Here's how the part is built. I have some questions about the finished solid (model axes, mm). Give positions to 0.01 mm unless a question says otherwise; leave off trailing zeros. Write each loop counter-clockwise with the first axis right and the second up, starting at its lowest first coordinate (ties: lowest second). Pieces come first, ordered by that corner, then holes. Notation, with made-up numbers: (58.5, 51.5) -> (73.5, 51.5) arc R21 cw to (73.5, 62.5) -> close; hole circle Ø10 at (64, 37). An arc over 180 degrees is marked (long way). Use one line per item in the form item = value.
Autodesk Inventor part; units mm, degrees
ref_plane "作業平面1" through (0, 8, 0) normal (0, -0.7881, 0.6155) x (1, 0, 0)
ref_plane "作業平面2" through (0, -5, -3.1241) normal (0, -0.977, 0.2132) x (-0.3818, -0.1971, -0.903)
ref_plane "作業平面3" through (-5, 8, -6) normal (0, 0, 1) x (1, 0, 0)
sketch "スケッチ1" plane through (0, 0, 0) normal (0, 1, 0) x (-1, 0, 0)
  line L0 (-17.5, -21) -> (0, 0)
  line L1 (0, 0) -> (17.5, -21)
  line L2 (17.5, -21) -> (17.5, -41)
  line L3 (17.5, -41) -> (0, -50)
  line L4 (0, -50) -> (-17.5, -41)
  line L5 (-17.5, -41) -> (-17.5, -21)
  line L6 (0, -60) -> (0, 10)
  line L7 (24.5, 0) -> (-24.5, 0)
  dimension "d0" = 50
  dimension "d12" = 35
  dimension "d13" = 20
  dimension "d14" = 21
extrude "押し出し1" add sketch "スケッチ1" along normal blind 18
chamfer "面取り1" distance 5 distance2 10 6 edges at (8.75, 18, -10.5) (17.5, 18, -31) (8.75, 18, -45.5) (-8.75, 18, -45.5) (-17.5, 18, -31) (-8.75, 18, -10.5) measured on face at (0, 18, -30.6667)
extrude "押し出し2" add sketch "スケッチ1" against normal blind 5
ref_plane "作業平面1" through (0, 8, 0) normal (0, -0.7881, 0.6155) x (1, 0, 0)
sketch "スケッチ2" plane through (0, 8, 0) normal (0, -0.7881, 0.6155) x (1, 0, 0)
  line L0 (0, 0) -> (17.5, -16.5503)
  line L1 (-17.5, -16.5503) -> (0, 0)
  line L2 (-5, -4.7287) -> (-5, -4.7287)
  line L3 (-5, -4.7287) -> (5, -4.7287)
  line L4 (13.3346, -12.611) -> (5, -4.7287)
  line L5 (-5, -4.7287) -> (-23.6413, -26.9446)
  line L6 (5, -4.7287) -> (18.7173, -21.0763)
  line L7 (-23.6413, -26.9446) -> (-26.2109, -24.7885)
  line L8 (-26.2109, -24.7885) -> (-17.5, -16.5503)
  line L9 (17.5, -16.5503) -> (23.8178, -21.8516)
  line L10 (23.8178, -21.8516) -> (18.7173, -21.0763)
  point P0 (0, -4.9243)
  dimension "d9" = 10
  dimension "d25" = 130
  dimension "d26" = 130
extrude "押し出し3" cut sketch "スケッチ2" against normal through all
chamfer "面取り2" distance 2 distance2 8 6 edges at (-8.75, -5, -10.5) (-17.5, -5, -31) (-8.75, -5, -45.5) (8.75, -5, -45.5) (17.5, -5, -31) (8.75, -5, -10.5) measured on face at (0, -5, -30.6667)
sketch "スケッチ3" plane through (0, -5, 0) normal (0, -1, 0) x (1, 0, 0)
  line L0 (0, -3.1241) -> (15.5, -21.7241)
  line L1 (-15.5, -21.7241) -> (0, -3.1241)
  line L2 (-15.5, -39.7796) -> (-15.5, -21.7241)
  line L3 (0, -47.751) -> (-15.5, -39.7796)
  line L4 (15.5, -39.7796) -> (0, -47.751)
  line L5 (15.5, -21.7241) -> (15.5, -39.7796)
  point P0 (0, 0)
extrude "押し出し4" add sketch "スケッチ3" along normal blind 8
ref_plane "作業平面2" through (0, -5, -3.1241) normal (0, -0.977, 0.2132) x (-0.3818, -0.1971, -0.903)
sketch "スケッチ4" plane through (0, -5, -3.1241) normal (0, -0.977, 0.2132) x (-0.3818, -0.1971, -0.903)
  line L0 (80, -28.4848) -> (-10, -28.4848)
  line L1 (-10, -28.4848) -> (-10, 40)
  line L2 (-10, 40) -> (80, 40)
  line L3 (80, 40) -> (80, -28.4848)
  point P0 (-3.8064, -1.5725)
extrude "押し出し5" cut sketch "スケッチ4" along normal through all
ref_plane "作業平面3" through (-5, 8, -6) normal (0, 0, 1) x (1, 0, 0)
sketch "スケッチ5" plane through (-5, 8, -6) normal (0, 0, 1) x (1, 0, 0)
  line L0 (-30, 20) -> (40, 20)
  line L1 (40, 20) -> (40, -30)
  line L2 (40, -30) -> (-30, -30)
  line L3 (-30, -30) -> (-30, 20)
  point P0 (5, -8)
extrude "押し出し6" cut sketch "スケッチ5" along normal through all
sketch "スケッチ6" plane through (-5, 8, -6) normal (0, 0, 1) x (1, 0, 0)
  line L0 (0, 0) -> (10, 0)
  circle A0 centre (5, 0) radius 5
  line L1 (9.9497, -4.9497) -> (5, -7)
  line L2 (5, -7) -> (0.0503, -4.9497)
  line L3 (0.0503, -4.9497) -> (-2, 0)
  line L4 (-2, 0) -> (0.0503, 4.9497)
  line L5 (0.0503, 4.9497) -> (5, 7)
  line L6 (5, 7) -> (9.9497, 4.9497)
  line L7 (9.9497, 4.9497) -> (12, 0)
  line L8 (12, 0) -> (9.9497, -4.9497)
  point P0 (5, -8)
  dimension "d29" = 7
extrude "押し出し7" cut sketch "スケッチ6" against normal blind 8 contours A0 L0 | L0 A0 | L1 L2 L3 L4 L5 L6 L7 L8
sketch "スケッチ8" plane through (-5, 8, -14) normal (0, 0, 1) x (1, 0, 0)
  line L0 (5, 0) -> (-12.5, 0)
  circle A0 centre (5, 0) radius 4
  line L1 (5, 4) -> (5, -4)
  line L2 (5, -5) -> (5, 0)
  point P0 (5, -8)
  dimension "d32" = 8
revolve "回転1" add sketch "スケッチ8" angle 360 about axis through (0, 12, -14) along (0, -1, 0) contours L1 A0
sketch "スケッチ9" plane through (-15.5, -5, -21.7241) normal (-0.7453, -0.2425, 0.6211) x (0.6214, 0.0849, 0.7789)
  circle A0 centre (10.2962, 6.6564) radius 0.8
  circle A1 centre (12.0048, 1.9574) radius 0.8
  circle A2 centre (7.081, 2.8272) radius 0.8
  circle A3 centre (2.1573, 3.697) radius 0.8
  circle A4 centre (5.3724, 7.5262) radius 0.8
  line L0 (2.1573, 3.697) -> (7.081, 2.8272) construction
  line L1 (7.081, 2.8272) -> (12.0048, 1.9574) construction
  line L2 (12.0048, 1.9574) -> (7.081, 2.8272)
  line L3 (5.3724, 7.5262) -> (10.2962, 6.6564) construction
  line L4 (10.2962, 6.6564) -> (9.5429, 2.3923) construction
  line L5 (5.3724, 7.5262) -> (4.6191, 3.2621) construction
  line L6 (10.2962, 6.6564) -> (12.0048, 1.9574) construction
  line L7 (12.0048, 1.9574) -> (11.7379, 0.4469) construction
  line L8 (12.0048, 1.9574) -> (13.2927, 2.4257) construction
  line L9 (20.3897, -1.7904) -> (19.4508, 6.57)
  line L10 (0, 0) -> (20.3897, -1.7904)
  point P0 (26.9765, 2.9875)
  dimension "d34" = 1.6
  dimension "d35" = 5
  dimension "d36" = 5
  dimension "d37" = 7.9143
  dimension "d38" = 3
extrude "押し出し8" cut sketch "スケッチ9" against normal blind 5
sketch "スケッチ10" plane through (-12.5, 18, -25.1515) normal (-0.766, 0.3957, 0.5066) x (0.5516, 0, 0.8341)
  circle A0 centre (2.1738, -2.388) radius 0.8
  circle A1 centre (0.2082, -6.8935) radius 0.8
  point P0 (27.8741, -17.8951)
extrude "押し出し9" cut sketch "スケッチ10" against normal blind 5
mirror "ミラー1" about plane through (0, 0, 0) normal (1, 0, 0) of "押し出し8", "押し出し9"
sketch "スケッチ11" plane through (0, -5, -3.1241) normal (0, -0.977, 0.2132) x (0.9242, -0.0814, -0.373)
  line L0 (3.339, -1.8055) -> (-1.091, -3.6357)
  line L1 (-7.0564, -23.5137) -> (-1.091, -3.6357)
  line L2 (0, -40.594) -> (-7.0564, -23.5137)
  line L3 (28.6512, -28.7573) -> (0, -40.594)
  line L4 (21.5948, -11.677) -> (28.6512, -28.7573)
  line L5 (3.339, -1.8055) -> (21.5948, -11.677)
  line L6 (0, -40.594) -> (21.5948, -11.677)
  line L7 (-7.0564, -23.5137) -> (28.6512, -28.7573)
  circle A0 centre (10.7974, -26.1355) radius 4.25
  point P0 (-1.5725, 3.8064)
  dimension "d43" = 8.5
ref_plane "作業平面4" through (0, -10.0527, -30.9651) normal (0, -0.977, 0.2132) x (1, 0, 0)
ref_plane "作業平面5" through (0, 16.5, 0) normal (0, 1, 0) x (1, 0, 0)
sketch "スケッチ15" plane through (0, 16.5, 0) normal (0, 1, 0) x (1, 0, 0)
  line L0 (-40, 60) -> (40, 60)
  line L1 (40, 60) -> (40, 0)
  line L2 (40, 0) -> (-40, 0)
  line L3 (-40, 0) -> (-40, 60)
  point P0 (0, 0)
extrude "押し出し15" cut sketch "スケッチ15" against normal through all
sketch "スケッチ16" plane through (0, 18, 0) normal (0, 1, 0) x (1, 0, 0)
  circle A0 centre (0, 41.8775) radius 0.8
  line L0 (-12.5, 37.949) -> (0, 44.3775)
  line L1 (-12.5, 25.1515) -> (-12.5, 37.949)
  line L2 (0, 44.3775) -> (12.5, 37.949)
  circle A1 centre (-10.2746, 36.8098) radius 0.8
  circle A2 centre (-10.2746, 26.2907) radius 0.8
  circle A3 centre (10.2746, 36.8098) radius 0.8
  circle A4 centre (10.2746, 26.2907) radius 0.8
  line L3 (0, 44.3775) -> (0, 41.0775) construction
  line L4 (12.5, 37.949) -> (9.5625, 36.4453) construction
  line L5 (-9.5625, 26.6552) -> (-12.5, 25.1515) construction
  line L6 (-12.5, 37.949) -> (-9.5625, 36.4453) construction
  line L7 (9.5625, 26.6552) -> (12.5, 25.1515) construction
  point P0 (0, 0)
  dimension "d65" = 1.6
  dimension "d66" = 1.6
  dimension "d67" = 1.6
  dimension "d68" = 1.6
  dimension "d69" = 1.6
  dimension "d70" = 2.5
extrude "押し出し16" cut sketch "スケッチ16" against normal through all
properties part number "head_bace_div_upper"
Q1. I want a section at B-B, the plane x = 5.75. Write out the boundary of the cut face in (y, z), and give its area (3 significant figures).
Result set:
outline = (16.5, -42.26) -> (18, -41.42) -> (18, -14.94) -> (16.5, -13.77) -> close
area = 41.2 mm2
Q2. I want a section at A-A, the plane y = 17.55. Count the separate pieces of the cut face and the enclosed holes in it, and give its area (3 significant figures).
Result set:
separate_pieces = 1
enclosed_holes = 5
area = 610 mm2
Q3. If we mould it in two halves opening along Z, with no side actions, what happens to faces 1 (the face through (9.475, 17.26, -26.326)), 2 (the face through (-6.549, 17.239, -41.437)), 3 (the face through (-8.801, 17.456, -19.132)), 4 (the face through (0, 18, -29))? For each: +Z half, -Z half, draft (parallel to the pull), parting line (faces both ways), or undercut.
Result set:
face_1 = undercut
face_2 = -Z half
face_3 = +Z half
face_4 = draft
Q4. Will this pin go through, and if not, where does the flat tip stop? pin 1 Ø2 at (x, z) = (0, -41.88) entering from +Y.
Result set:
pin_1 = 18
Q5. I want a section at C-C, the plane z = -15.5. Write out the boundary of the cut face in (x, y).
Result set:
outline = (-6.89, 16.5) -> (6.89, 16.5) -> (6.12, 18) -> (-6.12, 18) -> close
Q6. If I drill on line 1 along Z through (x, y) = (-10.5, 17.45); line 2 along Z through (x, y) = (-0.5, 16.95); line 3 along X through (y, z) = (17.85, -42), over which ranges is the centre line in solid material (lowest first)? Write a range as from..to.
Result set:
line_1 = -39.29..-37.58, -36.04..-27.06, -25.52..-21.7
line_2 = -44.71..-42.5, -41.25..-12.99
line_3 = -4.79..-0.79, 0.79..4.79
